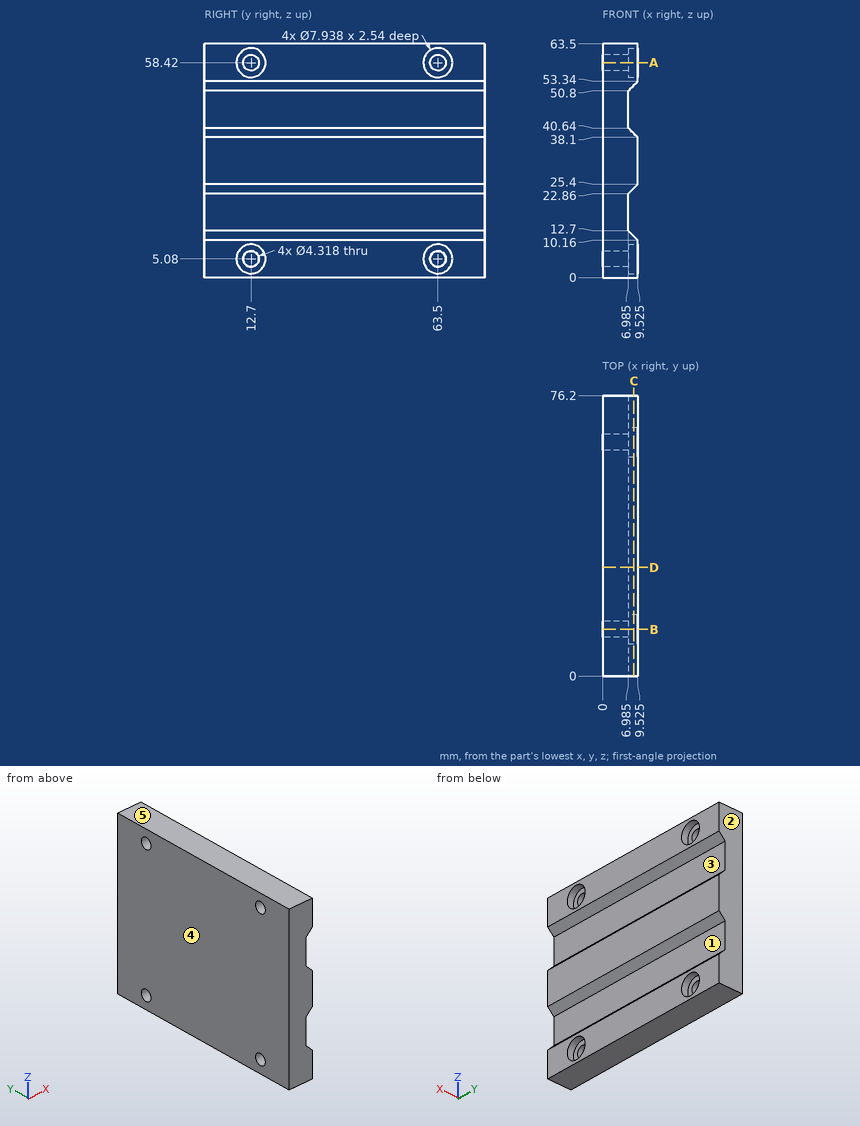
Source: three-view drawing plus pictorial views. Frame: mm from the lowest corner of the part. A direction names the side the tool comes from. Give positions to 0.01 mm unless a question says otherwise; leave off trailing zeros. Write each loop counter-clockwise with the first axis right and the second up, starting at its lowest first coordinate (ties: lowest second). Pieces come first, ordered by that corner, then holes.
(1) Mould query, pull axis Z, two halves, no side actions, for the marked faces 3, 4 and 5. Classes: released by +Z, released by -Z, zero draft, split by the parting line, or undercut.
(2) Cut plane C-C, the plane x = 8.5. Return loops of the section in (y, z) (1 decimal).
(3) Cut plane D-D, the plane y = 29.5. Return loops of the section in (x, z) (1 decimal).
(4) Cut plane B-B, the plane y = 12.7. Return loops of the section in (x, z) (1 decimal).
(5) Cut plane A-A, the plane z = 58.42. Return loops of the section in (x, y) (1 decimal), then the cut area to 3 significant figures.
(6) First-contact query: P1, Ø8, axis at y = 53, z = 18, coming from the +X side (1 decimal); P2, Ø8, axis at y = 26, z = 47, coming from the +X side (1 decimal). Flat tips, straight axial feed; report the tip coordinate or a pass-through.
(7) Access query for the marked faces 1 and 2. Directions: +Z, -Z, +X, -X, +Y, -Y. A direction counts if a zero-diameter tool reaches every point of the face in a straight line with its end or side. Return the directions, or none.
(8) Ray query, line 1 (Y direction, x = 5.5, z = 5.08); line 2 (Z direction, x = 3.5, y = 12.7); line 3 (Z direction, x = 9.25, y = 38) (1 decimal). Return the intervals inside material, ascending.
Values follow:
1. face 3: undercut
1. face 4: zero draft
1. face 5: released by +Z
2. outline: (0, 0) - (76.2, 0) - (76.2, 11.2) - (0, 11.2) - close; (0, 24.4) - (76.2, 24.4) - (76.2, 39.1) - (0, 39.1) - close; (0, 52.3) - (76.2, 52.3) - (76.2, 63.5) - (0, 63.5) - close; hole circle Ø7.9 at (12.7, 5.1); hole circle Ø7.9 at (12.7, 58.4); hole circle Ø7.9 at (63.5, 5.1); hole circle Ø7.9 at (63.5, 58.4)
3. outline: (0, 0) - (9.5, 0) - (9.5, 10.2) - (7, 12.7) - (7, 22.9) - (9.5, 25.4) - (9.5, 38.1) - (7, 40.6) - (7, 50.8) - (9.5, 53.3) - (9.5, 63.5) - (0, 63.5) - close
4. outline: (0, 0) - (9.5, 0) - (9.5, 1.1) - (7, 1.1) - (7, 2.9) - (0, 2.9) - close; (0, 7.2) - (7, 7.2) - (7, 9) - (9.5, 9) - (9.5, 10.2) - (7, 12.7) - (7, 22.9) - (9.5, 25.4) - (9.5, 38.1) - (7, 40.6) - (7, 50.8) - (9.5, 53.3) - (9.5, 54.5) - (7, 54.5) - (7, 56.3) - (0, 56.3) - close; (0, 60.6) - (7, 60.6) - (7, 62.4) - (9.5, 62.4) - (9.5, 63.5) - (0, 63.5) - close
5. outline: (0, 0) - (9.5, 0) - (9.5, 8.7) - (7, 8.7) - (7, 10.5) - (0, 10.5) - close; (0, 14.9) - (7, 14.9) - (7, 16.7) - (9.5, 16.7) - (9.5, 59.5) - (7, 59.5) - (7, 61.3) - (0, 61.3) - close; (0, 65.7) - (7, 65.7) - (7, 67.5) - (9.5, 67.5) - (9.5, 76.2) - (0, 76.2) - close
5. area: 625 mm2
6. P1: stops at x = 7
6. P2: stops at x = 7.2
7. face 1: +X, +Y, -Y
7. face 2: +Z, -Z, +X, -X, +Y
8. line 1: y = 0 to 10.54, 14.86 to 61.34, 65.66 to 76.2
8. line 2: z = 0 to 2.92, 7.24 to 56.26, 60.58 to 63.5
8. line 3: z = 0 to 10.4, 25.1 to 38.4, 53.1 to 63.5
